```python
from build123d import *

# Parameters (mm, degrees)
SKETCH1_R           = 12.5
SKETCH1_R_2         = 1.25
BOSS_EXTRUDE1_DEPTH = 53.5
SKETCH2_R           = 3.5
BOSS_EXTRUDE2_DEPTH = 2.5
BOSS_EXTRUDE3_DEPTH = 10.5


with BuildPart() as part:
    # Sketch1 → Boss-Extrude1 (new body)
    with BuildSketch(Plane.XY):
        Circle(SKETCH1_R)
        with Locations((-8.5, 0)):
            Circle(SKETCH1_R_2, mode=Mode.SUBTRACT)
        with Locations((8.5, 0)):
            Circle(SKETCH1_R_2, mode=Mode.SUBTRACT)
    extrude(amount=BOSS_EXTRUDE1_DEPTH)

    # Sketch2 → Boss-Extrude2 (add)
    with BuildSketch(Plane.XY.offset(53.5)):
        Circle(SKETCH2_R)
    extrude(amount=BOSS_EXTRUDE2_DEPTH)

    # Sketch3 → Boss-Extrude3 (add)
    with BuildSketch(Plane.XY.offset(56)):
        with BuildLine():
            Line((-1.2, 1.6), (1.2, 1.6))
            ThreePointArc((1.2, 1.6), (0, -2), (-1.2, 1.6))
        make_face()
    extrude(amount=BOSS_EXTRUDE3_DEPTH)


solid = part.part
```
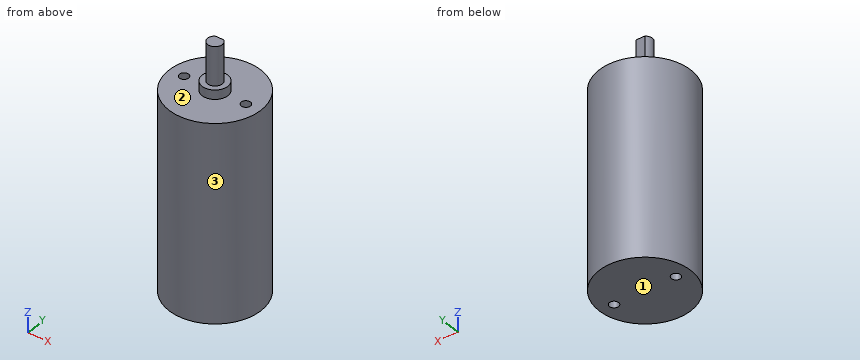
Geometry check sheet. Reference: the model listing, model coordinates, mm. Face numbers are marked on the shaded views. Round coordinates to 2 decimals unless told otherwise and drop trailing zeros. Order: outer loops, then holes, each group sorted by start corner. A loop starts at its lowest first (then second) coordinate and runs counter-clockwise, first axis right, second up. Notation, with made-up numbers: (85, 52.25) - (97, 52.25) arc R10 cw to (97, 67.25) - close; hole circle Ø3 at (54.5, 77.5). An arc over 180 degrees is marked (long way). Use a Markdown table: item, result. Add a question column.
1) Section check C-C (x = 0). Record the cut outline in (y, z).
2) Thickness scan on line 1 along X through (y, z) = (-1, 9); line 2 along Z through (x, y) = (4.25, -1.5); line 3 along Y through (x, z) = (-8.5, 35.5). Record the ranges inside material, lowest first.
3) Section check D-D (z = 29). Record the cut outline in (x, y), then the cut area to 3 significant figures.
4) Section check A-A (y = 0). Record the cut outline in (x, z).
5) Gauge pin test, flat ends, axial feed: P1, Ø1.5, axis at x = 8.5, y = 0, coming from the +Z side; P2, Ø3, axis at x = 6.5, z = 33, coming from the -Y side; P3, Ø4, axis at x = 7.5, z = 46, coming from the +Y side (3 decimals); P4, Ø5, axis at x = 6, z = 13.5, coming from the -Y side. Record the tip position at first contact, or that the pin passes through.
6) Mould release check, pull along Z, two halves, no side actions. Record for the marked faces 1, 2 and 3: released by +Z, released by -Z, zero draft, split by the parting line, or undercut.
7) Section check B-B (x = -8). Record the cut outline in (y, z), then the cut area to 3 significant figures.
Established:
| question | item | result |
|---|---|---|
| 1 | outline | (-12.5, 0) - (12.5, 0) - (12.5, 53.5) - (3.5, 53.5) - (3.5, 56) - (1.6, 56) - (1.6, 66.5) - (-2, 66.5) - (-2, 56) - (-3.5, 56) - (-3.5, 53.5) - (-12.5, 53.5) - close |
| 2 | line 1 | -12.46 to -9.25, -7.75 to 7.75, 9.25 to 12.46 |
| 2 | line 2 | 0 to 53.5 |
| 2 | line 3 | -9.17 to -1.25, 1.25 to 9.17 |
| 3 | outline | circle Ø25 at (0, 0); hole circle Ø2.5 at (-8.5, 0); hole circle Ø2.5 at (8.5, 0) |
| 3 | area | 481 mm2 |
| 4 | outline | (-12.5, 0) - (-9.75, 0) - (-9.75, 53.5) - (-12.5, 53.5) - close; (-7.25, 0) - (7.25, 0) - (7.25, 53.5) - (3.5, 53.5) - (3.5, 56) - (2, 56) - (2, 66.5) - (-2, 66.5) - (-2, 56) - (-3.5, 56) - (-3.5, 53.5) - (-7.25, 53.5) - close; (9.75, 0) - (12.5, 0) - (12.5, 53.5) - (9.75, 53.5) - close |
| 5 | P1 | through |
| 5 | P2 | y = -11.46 |
| 5 | P3 | y = 11.225 |
| 5 | P4 | y = -12 |
| 6 | face 1 | released by -Z |
| 6 | face 2 | released by +Z |
| 6 | face 3 | zero draft |
| 7 | outline | (-9.6, 0) - (-1.15, 0) - (-1.15, 53.5) - (-9.6, 53.5) - close; (1.15, 0) - (9.6, 0) - (9.6, 53.5) - (1.15, 53.5) - close |
| 7 | area | 905 mm2 |
